The model under review builds one solid part; all positions refer to its coordinate system, in mm. Face numbers are marked on the shaded views. A direction names the side the tool comes from. Coordinates: 2 decimals unless noted, no trailing zeros. Order: outer loops, then holes, each group sorted by start corner. A loop starts at its lowest first (then second) coordinate and runs counter-clockwise, first axis right, second up.
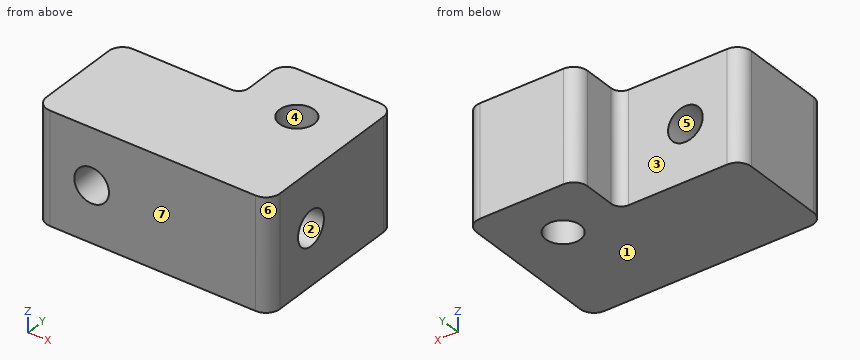
Autodesk Inventor part; units mm, degrees
ref_plane "YZ Plane" through (0, 0, 0) normal (1, 0, 0) x (0, 1, 0)
ref_plane "XZ Plane" through (0, 0, 0) normal (0, 1, 0) x (-1, 0, 0)
ref_plane "XY Plane" through (0, 0, 0) normal (0, 0, 1) x (1, 0, 0)
sketch "Sketch1" plane through (0, 0, 0) normal (0, 0, 1) x (1, 0, 0)
  line L0 (6.35, -9.525) -> (-6.35, -9.525)
  line L1 (-6.35, 3.175) -> (-6.35, 9.525)
  line L2 (-6.35, 9.525) -> (6.35, 9.525)
  line L3 (6.35, 9.525) -> (6.35, -9.525)
  line L4 (6.35, -9.525) -> (-6.35, 9.525) construction
  line L5 (-6.35, -9.525) -> (6.35, 9.525) construction
  line L6 (-6.35, -9.525) -> (-20.32, -9.525)
  line L7 (-20.32, -9.525) -> (-20.32, 3.175)
  line L8 (-20.32, 3.175) -> (-6.35, 3.175)
  line L9 (-6.35, 3.175) -> (-6.35, -9.525) construction
  point P0 (0, 0)
  dimension "d0" = 12.7
  dimension "d1" = 19.05
  dimension "d3" = 12.7
  dimension "d4" = 13.97
extrude "Plate1" add sketch "Sketch1" along normal blind 12.7
sketch "Sketch2" plane through (0, 0, 12.7) normal (0, 0, 1) x (1, 0, 0)
  line L0 (-6.35, 9.525) -> (6.35, 9.525)
  point P0 (0, 0)
  point P1 (0, 3.175)
  dimension "d5" = 6.35
hole "Hole1" at (0, 3.175, 12.7) direction (0, 0, -1) diameter 3.9624 depth 13.6144 tip angle 118
sketch "Sketch3" plane through (-20.32, -9.525, 0) normal (0, -1, 0) x (1, 0, 0)
  line L0 (0, 0) -> (0, 12.7)
  line L1 (0, 0) -> (26.67, 0)
  point P0 (20.32, 0)
  point P1 (6.35, 6.35)
  dimension "d13" = 6.35
  dimension "d14" = 6.35
hole "Hole2" at (-13.97, -9.525, 6.35) direction (0, 1, 0) diameter 3.9624 depth 23.1394 tip angle 118
sketch "Sketch4" plane through (6.35, -9.525, 0) normal (1, 0, 0) x (0, 0, -1)
  line L0 (0, 0) -> (-12.7, 0)
  line L1 (-12.7, 19.05) -> (-12.7, 0)
  point P0 (0, 9.525)
  point P1 (-6.35, 6.35)
  dimension "d22" = 6.35
  dimension "d23" = 6.35
hole "Hole3" at (6.35, -3.175, 6.35) direction (-1, 0, 0) diameter 3.9624 depth 12.7 tip angle 118
fillet "Corner Round1" radius 1.5875 5 edges at (6.35, 9.525, 6.35) (-6.35, 9.525, 6.35) (-20.32, 3.175, 6.35) (-20.32, -9.525, 6.35) (6.35, -9.525, 6.35)
fillet "Corner Round1" radius 1.143 1 edges at (-6.35, 3.175, 6.35)
equation "\"d29\" = Thickness"
equation "\"d2\" = Thickness"
equation "\"BendRadius\" = Thickness"
equation "\"BendReliefWidth\" = Thickness"
equation "\"BendReliefDepth\" = 0.5 * Thickness"
equation "\"CornerReliefSize\" = 4 * Thickness"
equation "\"MinimumRemnant\" = 2 * Thickness"
equation "\"TransitionRadius\" = BendRadius"
equation "\"JacobiRadiusSize\" = BendRadius"
equation "\"GapSize\" = Thickness"
properties part number "PLATE,NUT-BLOCK,L-SHAPE" material "Aluminum 6061"
(1) Insertion check: pin 1 Ø4 at (y, z) = (5.5, 5.5) entering from -X; pin 2 Ø3.5 at (x, z) = (-12.5, 8.5) entering from +Y (3 decimals); pin 3 Ø5 at (x, z) = (-13.97, 6.35) entering from -Y (3 decimals); pin 4 Ø2 at (y, z) = (3, 10) entering from -X. Each pin has a flat end and moves straight along its axis. Give the tip position at first contact, or say it passes through.
(2) Consider section A-A (x = -0.75). Give the boundary of the cut face in (y, z) (3 decimals).
(3) Consider section D-D (z = 5.25). Give the number of separate pieces and of enclosed holes in the cut face, then the cut area to 3 significant figures.
(4) Consider section C-C (x = -13.97). Give the boundary of the cut face in (y, z) (3 decimals).
(5) Wall thickness on line 1 (Y direction, x = -2.25, z = 6.35) (3 decimals); line 2 (Y direction, x = 0, z = 3) (3 decimals); line 3 (Z direction, x = -13.97, y = -1.5): over which ranges is each line inside the solid? List them lowest first.
(6) The part is to be moulded in two halves that separate along X. For the marked faces 4, 5, 6 and 7, say which applies: +X half, -X half, draft (parallel to the pull), parting line (faces both ways), or undercut.
(7) Tool access review of the marked faces 1, 2 and 3: name each direction out of +Z, -Z, +X, -X, +Y, -Y from which nothing blocks a thin tool from reaching the whole face with its end or side.
Findings:
1. pin 1: stops at x = -6.69
1. pin 2: stops at y = 3.175
1. pin 3: stops at y = -9.525
1. pin 4: stops at x = -20.27
2. outline: (-9.525, 0) - (1.341, 0) - (1.341, 12.7) - (-9.525, 12.7) - close; (5.009, 0) - (9.525, 0) - (9.525, 12.7) - (5.009, 12.7) - close; hole circle Ø3.962 at (-3.175, 6.35)
3. separate pieces: 2
3. enclosed holes: 1
3. area: 320 mm2
4. outline: (-9.525, 0) - (3.175, 0) - (3.175, 4.369) - (-9.525, 4.369) - close; (-9.525, 8.331) - (3.175, 8.331) - (3.175, 12.7) - (-9.525, 12.7) - close
5. line 1: y = -9.525 to -5.156, -1.194 to 9.525
5. line 2: y = -9.525 to 1.194, 5.156 to 9.525
5. line 3: z = 0 to 4.37, 8.33 to 12.7
6. face 4: undercut
6. face 5: undercut
6. face 6: +X half
6. face 7: draft
7. face 1: -Z, +X, -X, +Y, -Y
7. face 2: +X
7. face 3: +Z, -Z, -X, +Y
